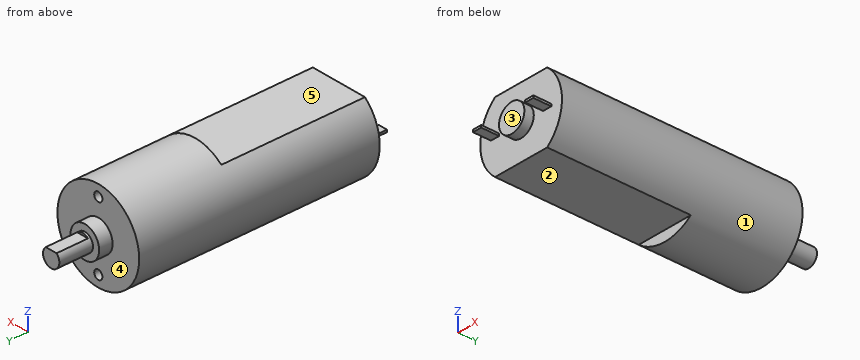
Autodesk Inventor part; units mm, degrees
ref_plane "YZ Plane" through (0, 0, 0) normal (1, 0, 0) x (0, 1, 0)
ref_plane "XZ Plane" through (0, 0, 0) normal (0, 1, 0) x (-1, 0, 0)
ref_plane "XY Plane" through (0, 0, 0) normal (0, 0, 1) x (1, 0, 0)
sketch "Эскиз1" plane through (0, 0, 0) normal (0, 1, 0) x (-1, 0, 0)
  circle A0 centre (0, 0) radius 10
  circle A1 centre (0, 0) radius 3.5
  circle A2 centre (0, 0) radius 2
  dimension "d0" = 20
  dimension "d1" = 7
  dimension "d2" = 4
extrude "Выдавливание1" add sketch "Эскиз1" against normal blind 21.6 contours A0 | A1 | A2
extrude "Выдавливание2" add sketch "Эскиз1" along normal blind 3 contours A1
extrude "Выдавливание3" add sketch "Эскиз1" along normal blind 10.5 contours A2
sketch "Эскиз2" plane through (0, 10.5, 0) normal (0, 1, 0) x (1, 0, 0)
  circle A0 centre (0, 0) radius 2
  circle A1 centre (0, 0) radius 2
  circle A2 centre (0, 0) radius 3.5
  line L0 (-3.1623, -1.5) -> (3.1623, -1.5)
  point P0 (0, 2)
  point P1 (0, 3.5)
  point P2 (1.3229, -1.5)
  point P3 (-1.3229, -1.5)
  dimension "d9" = 1.5
extrude "Выдавливание4" cut sketch "Эскиз2" against normal blind 7 contours L0 A0 picked at (0.3089, -1.5908)
sketch "Эскиз3" plane through (0, -21.6, 0) normal (0, -1, 0) x (1, 0, 0)
  line L0 (6.3804, -7.7) -> (-6.3804, -7.7)
  line L1 (-6.3804, -7.7) -> (-6.3804, 7.7)
  line L2 (-6.3804, 7.7) -> (6.3804, 7.7)
  line L3 (6.3804, 7.7) -> (6.3804, -7.7)
  circle A0 centre (0, 0) radius 10
  arc A1 (6.3804, -7.7) -> (6.3804, 7.7) centre (0, 0) ccw
  arc A2 (-6.3804, 7.7) -> (-6.3804, -7.7) centre (0, 0) ccw
  line L4 (5.3804, 0.25) -> (7.3804, 0.25)
  line L5 (7.3804, 0.25) -> (7.3804, -0.25)
  line L6 (7.3804, -0.25) -> (5.3804, -0.25)
  line L7 (5.3804, -0.25) -> (5.3804, 0.25)
  line L8 (5.3804, 0.25) -> (7.3804, -0.25) construction
  line L9 (0, -7.7) -> (0, 7.7) construction
  line L10 (-5.3804, 0.25) -> (-7.3804, 0.25)
  line L11 (-7.3804, 0.25) -> (-7.3804, -0.25)
  line L12 (-7.3804, -0.25) -> (-5.3804, -0.25)
  line L13 (-5.3804, -0.25) -> (-5.3804, 0.25)
  point P0 (6.3804, 0)
  point P1 (-6.3804, -7.7)
  dimension "d12" = 15.4
  dimension "d13" = 2
  dimension "d14" = 0.5
extrude "Выдавливание5" add sketch "Эскиз3" along normal blind 36 contours L6 L7 L4 L3 | L3 L4 L5 L6 | L12 L11 L10 L1 | L1 L10 L13 L12
extrude "Выдавливание6" add sketch "Эскиз3" along normal blind 32 contours L0 L1 L12 L13 L10 L2 L3 L4 L7 L6 | L3 L6 L5 L4 A0 | A0 L1 L10 L11 L12
sketch "Эскиз4" plane through (0, -53.6, 0) normal (0, -1, 0) x (1, 0, 0)
  circle A0 centre (0, 0) radius 2
  circle A1 centre (0, 0) radius 3.1
  dimension "d19" = 6.2
extrude "Выдавливание7" add sketch "Эскиз4" along normal blind 2.1 contours A0 | A1
sketch "Эскиз5" plane through (0, 0, 0) normal (0, 1, 0) x (1, 0, 0)
  circle A0 centre (0, 0) radius 10 construction
  line L0 (0, 10) -> (0, -10) construction
  circle A1 centre (0, 7.5) radius 1
  circle A2 centre (0, -7.5) radius 1
  dimension "d22" = 7.5
  dimension "d23" = 15
  dimension "d24" = 2
hole "Отверстие1" at (0, 0, 7.5) direction (0, -1, 0) diameter 2 depth 8 tip angle 118
hole "Отверстие2" at (0, 0, -7.5) direction (0, -1, 0) diameter 2 depth 8 tip angle 118
properties part number "motor20" material "Сталь"
Could you check a few things on this model? Use its own coordinates, in mm. Face numbers are marked on the shaded views. A direction names the side the tool comes from. Give positions to 0.01 mm unless a question says otherwise; leave off trailing zeros. Order: outer loops, then holes, each group sorted by start corner. A loop starts at its lowest first (then second) coordinate and runs counter-clockwise, first axis right, second up. Notation, with made-up numbers: (41.5, 75) -> (93.5, 75) arc R18 ccw to (93.5, 86) -> close; hole circle Ø4 at (-32.5, 25). An arc over 180 degrees is marked (long way). Return JSON: item names as keys, results as strings.
1. Imagine slicing it at A-A on y = -35. List the corners of the cut face in (x, z) for me, then the cut area to 3 significant figures.
Answer list:
{"outline": "(-6.38, -7.7) -> (6.38, -7.7) arc R10 ccw to (6.38, 7.7) -> (-6.38, 7.7) arc R10 ccw to start", "area": "274 mm2"}
2. Imagine slicing it at B-B on y = -6.5. List the corners of the cut face in (x, z) for me, then the cut area to 3 significant figures.
Answer list:
{"outline": "circle Ø20 at (0, 0); hole circle Ø2 at (0, -7.5); hole circle Ø2 at (0, 7.5)", "area": "308 mm2"}
3. For pin 1 Ø1.3 at (x, y) = (0.5, 8) entering from +Z; pin 2 Ø10 at (x, y) = (-2, -13.5) entering from -Z; pin 3 Ø5 at (y, z) = (-6, 6.5) entering from -X; pin 4 Ø8 at (x, y) = (-6, -38.5) entering from +Z, each with a flat end and sliding along its axis, tell me the tip position at first contact or that it passes through.
Answer list:
{"pin 1": "stops at z = 1.5", "pin 2": "stops at z = -10", "pin 3": "stops at x = -9.17", "pin 4": "stops at z = 7.7"}
4. On a 3-axis mill with a long thin cutter (end or side, diameter ignored), from which of +Z, -Z, +X, -X, +Y, -Y can I reach the whole of each face in a straight line? I mean the marked faces 4 and 5. Say none if no direction works.
Answer list:
{"face 4": "+Y", "face 5": "+Z, +X, -X, -Y"}
5. Imagine slicing it at C-C on x = 8.5. List the corners of the cut face in (y, z) for me.
Answer list:
{"outline": "(-53.6, -5.27) -> (0, -5.27) -> (0, 5.27) -> (-53.6, 5.27) -> close"}
6. I need wall thicknesses on line 1 (Z direction, x = 0, y = -3); line 2 (Y direction, x = 9, z = -4); line 3 (X direction, y = -5.75, z = 7.5). Which ranges of each line are inside material? Lowest first, please. Write a range as from..to.
Answer list:
{"line 1": "z = -10..-8.5, -6.5..6.5, 8.5..10", "line 2": "y = -53.6..0", "line 3": "x = -6.61..-1, 1..6.61"}
7. Thinking about a two-plate mould opening in X: for the marked faces 1, 2 and 3, which applies, pulls with the +X half, pulls with the -X half, needs draft (parallel to the pull), parting line crosses it, or undercut?
Answer list:
{"face 1": "parting line crosses it", "face 2": "needs draft", "face 3": "undercut"}
